Work out the finished part from the listing and answer in its coordinate system (mm). A direction names the side the tool comes from. Round coordinates to 2 decimals unless told otherwise and drop trailing zeros. Write each loop counter-clockwise with the first axis right and the second up, starting at its lowest first coordinate (ties: lowest second). Pieces come first, ordered by that corner, then holes.
from build123d import *

# Parameters (mm, degrees)
SKETCH1_R                = 3.5
BOSS_EXTRUDE1_DEPTH      = 4
SKETCH2_R                = 2.5
BOSS_EXTRUDE2_DEPTH      = 50
BOSS_EXTRUDE3_DEPTH      = 2
BOSS_EXTRUDE3_DEPTH_BACK = 2


with BuildPart() as part:
    # Sketch1 → Boss-Extrude1 (new body)
    with BuildSketch(Plane.XY):
        with BuildLine():
            Line((0, -3), (-70.390227771, -3))
            ThreePointArc((-70.390227771, -3), (-80.5, 0), (-70.390227771, 3))
            Line((-70.390227771, 3), (0, 3))
            ThreePointArc((0, 3), (3, 0), (0, -3))
        make_face()
        with Locations((-75, 0)):
            Circle(SKETCH1_R, mode=Mode.SUBTRACT)
    extrude(amount=BOSS_EXTRUDE1_DEPTH)

    # Sketch2 → Boss-Extrude2 (add)
    with BuildSketch(Plane.XY.offset(4)):
        Circle(SKETCH2_R)
    extrude(amount=BOSS_EXTRUDE2_DEPTH)

    # Sketch3 → Boss-Extrude3 (add, two sides)
    with BuildSketch(Plane(origin=(0, 0, 0), x_dir=(1, 0, 0), z_dir=(0, 1, 0))) as boss_extrude3_sk:
        Polygon((-22.626919406, -2.400081024), (-16.082292112, -2.400081024), (0, -14.514826908), (0, -21.639035848), align=None)
    extrude(amount=BOSS_EXTRUDE3_DEPTH)
    extrude(boss_extrude3_sk.sketch, amount=-BOSS_EXTRUDE3_DEPTH_BACK)


solid = part.part
Q1. The mould has two halves that part along Y. Classify faces 1 (the face through (-9, 2, 10)), 2 (the face through (-71.767, -1.341, 1.972)), 3 (the face through (-38, 0, 4)), 4 (the face through (3, 0, 2)): +Y half, -Y half, draft (parallel to the pull), parting line (faces both ways), or undercut.
Q2. Given pin 1 (8 mm diameter, centred on x = -12.5, z = 10, fed in from +Y); pin 2 (5 mm diameter, centred on y = -4.5, z = 37, fed in from +X); pin 3 (4 mm diameter, centred on x = -11.5, y = -1, fed in from -Z); pin 4 (4 mm diameter, centred on x = -71.5, y = 4, fed in from +Z), each flat-ended and moving along its own axis, determine where each tip first touches the part or whether it passes through.
Q3. A tool of negligible diameter and unlimited length cuts with its end or side. For faces 5 (the face through (-36, 3, 2)), 6 (the face through (-35, -3, 2)), 7 (the face through (-9, -2, 10)), from which of +Z, -Z, +X, -X, +Y, -Y can it reach the whole face along a straight path? Write none if from no direction.
Q4. Find section A-A (y = 0). Determine the outline of the cut face in (x, z).
Q5. Find section D-D (x = -48). Determine the outline of the cut face in (y, z), plus the area to 3 significant figures.
Q6. Find section B-B (x = -75). Determine the outline of the cut face in (y, z), plus the area to 3 significant figures.
Q7. Find section C-C (z = 22). Determine the outline of the cut face in (x, y).
Q8. Find the intervals of material crossed by L1, parallel to Y at x = -75, z = 2; L2, parallel to X at y = 1.5, z = 48; L3, parallel to X at y = -2, z = 3.5, in increasing order.
Report:
1. face 1: +Y half
1. face 2: undercut
1. face 3: draft
1. face 4: parting line
2. pin 1: stops at y = 2
2. pin 2: stops at x = 1.5
2. pin 3: stops at z = 0
2. pin 4: stops at z = 4
3. face 5: +Z, -Z, +X, +Y
3. face 6: +Z, -Z, +X, -Y
3. face 7: +Z, -X, -Y
4. outline: (-80.5, 0) - (-78.5, 0) - (-78.5, 4) - (-80.5, 4) - close; (-71.5, 0) - (3, 0) - (3, 4) - (2.5, 4) - (2.5, 54) - (-2.5, 54) - (-2.5, 19.51) - (-20.75, 4) - (-71.5, 4) - close; hole (-13.96, 4) - (-2.5, 4) - (-2.5, 12.63) - close
5. outline: (-3, 0) - (3, 0) - (3, 4) - (-3, 4) - close
5. area: 24.0 mm2
6. outline: (-5.5, 0) - (-3.5, 0) - (-3.5, 4) - (-5.5, 4) - close; (3.5, 0) - (5.5, 0) - (5.5, 4) - (3.5, 4) - close
6. area: 16.0 mm2
7. outline: circle Ø5 at (0, 0)
8. L1: y = -5.5 to -3.5, 3.5 to 5.5
8. L2: x = -2 to 2
8. L3: x = -80.12 to -77.87, -72.13 to 2.24
